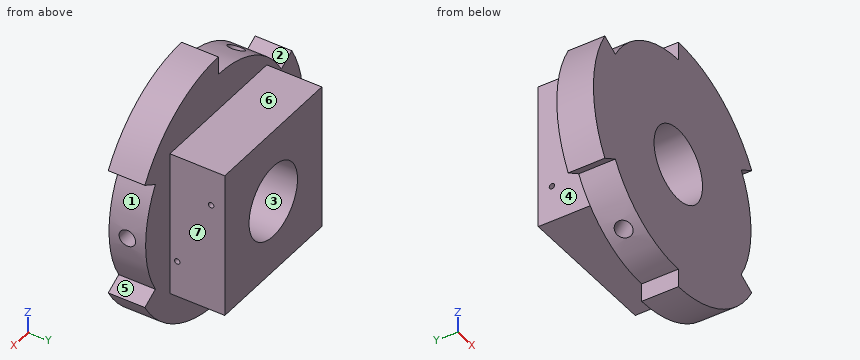
```python
from build123d import *

# Parameters (mm, degrees)
SKETCH1_R           = 30
BOSS_EXTRUDE3_DEPTH = 10
SKETCH2_R           = 2.25
CUT_EXTRUDE1_DEPTH  = 25
CIRPATTERN1_COUNT   = 3
SKETCH3_W           = 40
SKETCH3_H           = 40
BOSS_EXTRUDE4_DEPTH = 15
SKETCH5_R           = 10
CUT_EXTRUDE5_DEPTH  = 25
SKETCH4_R           = 0.75
CUT_EXTRUDE6_DEPTH  = 6
CIRPATTERN2_COUNT   = 2


with BuildPart() as part:
    # Sketch1 → Boss-Extrude3 (new body)
    with BuildSketch(Plane(origin=(0, 0, 0), x_dir=(1, 0, 0), z_dir=(0, 1, 0))):
        with BuildLine():
            Line((-25.980762114, 15), (-30.310889132, 17.5))
            ThreePointArc((-30.310889132, 17.5), (-35, 0), (-30.310889132, -17.5))
            Line((-30.310889132, -17.5), (-25.980762114, -15))
            ThreePointArc((-25.980762114, -15), (-30, 0), (-25.980762114, 15))
        make_face()
        Circle(SKETCH1_R)
        with BuildLine():
            Line((0, 35), (0, 30))
            ThreePointArc((0, 30), (15, 25.980762114), (25.980762114, 15))
            Line((25.980762114, 15), (30.310889132, 17.5))
            ThreePointArc((30.310889132, 17.5), (17.5, 30.310889132), (0, 35))
        make_face()
        with BuildLine():
            ThreePointArc((25.980762114, -15), (15, -25.980762114), (0, -30))
            Line((0, -30), (0, -35))
            ThreePointArc((0, -35), (17.5, -30.310889132), (30.310889132, -17.5))
            Line((30.310889132, -17.5), (25.980762114, -15))
        make_face()
    extrude(amount=BOSS_EXTRUDE3_DEPTH)

    # Sketch2 → Cut-Extrude1 (cut)
    with BuildSketch(Plane(origin=(40, 0, 0), x_dir=(0, 0, -1), z_dir=(1, 0, 0))):
        with Locations((0, 5)):
            Circle(SKETCH2_R)
    cut_extrude1 = extrude(amount=-CUT_EXTRUDE1_DEPTH, mode=Mode.SUBTRACT)

    # CirPattern1: Cut-Extrude1 ×3 about axis
    cirpattern1_axis = Axis((0, 0, 0), (0, 1, 0))
    for i in range(1, CIRPATTERN1_COUNT):
        add(cut_extrude1.rotate(cirpattern1_axis, i * 360 / CIRPATTERN1_COUNT), mode=Mode.SUBTRACT)

    # Sketch3 → Boss-Extrude4 (add)
    with BuildSketch(Plane(origin=(0, 10, 0), x_dir=(1, 0, 0), z_dir=(0, 1, 0))):
        Rectangle(SKETCH3_W, SKETCH3_H)
    extrude(amount=BOSS_EXTRUDE4_DEPTH)

    # Sketch5 → Cut-Extrude5 (cut)
    with BuildSketch(Plane(origin=(0, 25, 0), x_dir=(1, 0, 0), z_dir=(0, 1, 0))):
        with Locations(Location((0, 0, 0), (0, 0, 270))):
            Circle(SKETCH5_R)
    extrude(amount=-CUT_EXTRUDE5_DEPTH, mode=Mode.SUBTRACT)

    # Sketch4 → Cut-Extrude6 (cut)
    with BuildSketch(Plane(origin=(20, 0, 0), x_dir=(0, 0, -1), z_dir=(1, 0, 0))):
        with Locations((-10, 21.25)):
            Circle(SKETCH4_R)
        with Locations((10, 12)):
            Circle(SKETCH4_R)
    cut_extrude6 = extrude(amount=-CUT_EXTRUDE6_DEPTH, mode=Mode.SUBTRACT)

    # CirPattern2: Cut-Extrude6 ×2 about axis
    cirpattern2_axis = Axis((0, -28.284271247, 0), (0, 1, 0))
    for i in range(1, CIRPATTERN2_COUNT):
        add(cut_extrude6.rotate(cirpattern2_axis, i * 360 / CIRPATTERN2_COUNT), mode=Mode.SUBTRACT)


solid = part.part
```
Here's how the part is built. I have some questions about the finished solid (model axes, mm). Face numbers are marked on the shaded views. A direction names the side the tool comes from. Give positions to 0.01 mm unless a question says otherwise; leave off trailing zeros. Order: outer loops, then holes, each group sorted by start corner. A loop starts at its lowest first (then second) coordinate and runs counter-clockwise, first axis right, second up. Notation, with made-up numbers: M -13,1.25 L 3,1.25 A9 cw 3,8.25 Z; hole C 35,88.25 d7. An arc over 180 degrees is marked long. Use a Markdown table: item, result. Add a question column.
1. I need wall thicknesses on probe 1 along Y at (x, z) = (-17.15, 10); probe 2 along X at (y, z) = (14.75, 0); probe 3 along X at (y, z) = (3.5, -16). Which ranges of each line are inside material? Lowest first, please. Write a range as from..to.
2. If we mould it in two halves opening along Z, with no side actions, what happens to the marked faces 1, 2, 3 and 4? For each: +Z half, -Z half, draft (parallel to the pull), parting line (faces both ways), or undercut.
3. Suppose I cut it at C-C (x = -3). List the corners of the cut face in (y, z) for me, and give its area (3 significant figures).
4. Suppose I cut it at D-D (z = 16). Give the number of separate pieces and of enclosed holes in the cut face, and give its area (3 significant figures).
5. Suppose I cut it at A-A (z = 0). List the corners of the cut face in (x, y) for me.
6. For pin 1 Ø10 at (x, z) = (7, 16) entering from -Y; pin 2 Ø3.5 at (y, z) = (5, 0) entering from +X; pin 3 Ø12 at (x, y) = (-7.5, 20.5) entering from -Z; pin 4 Ø7.5 at (y, z) = (21, 5) entering from +X, each with a flat end and sliding along its axis, tell me the tip position at first contact or that it passes through.
7. Suppose I cut it at B-B (y = 17.25). List the corners of the cut face in (x, z) for me, and give its area (3 significant figures).
8. On a 3-axis mill with a long thin cutter (end or side, diameter ignored), from which of +Z, -Z, +X, -X, +Y, -Y can I reach the whole of each face in a straight line? I mean the marked faces 5, 6 and 7. Say none if no direction works.
Results list:
| question | item | result |
|---|---|---|
| 1 | probe 1 | y = 0..11.25, 12.75..25 |
| 1 | probe 2 | x = -20..-10, 10..20 |
| 1 | probe 3 | x = -31.13..-27.71, -25.38..-11.17, -7.3..27.71 |
| 2 | face 1 | undercut |
| 2 | face 2 | +Z half |
| 2 | face 3 | undercut |
| 2 | face 4 | draft |
| 3 | outline | M 0,-29.85 L 10,-29.85 L 10,-20 L 25,-20 L 25,-9.54 L 0,-9.54 Z; M 0,9.54 L 25,9.54 L 25,20 L 10,20 L 10,29.85 L 0,29.85 Z |
| 3 | area | 720 mm² |
| 4 | separate pieces | 2 |
| 4 | enclosed holes | 1 |
| 4 | area | 1,150 mm² |
| 5 | outline | M -35,0 L -10,0 L -10,25 L -20,25 L -20,10 L -35,10 Z; M 10,0 L 30,0 L 30,2.75 L 15,2.75 L 15,7.25 L 30,7.25 L 30,10 L 20,10 L 20,25 L 10,25 Z |
| 6 | pin 1 | stops at y = 0 |
| 6 | pin 2 | stops at x = 15 |
| 6 | pin 3 | stops at z = -20 |
| 6 | pin 4 | stops at x = 20 |
| 7 | outline | M -20,-20 L 20,-20 L 20,20 L -20,20 Z; hole C 0,0 d20 |
| 7 | area | 1,290 mm² |
| 8 | face 5 | +X, +Y, -Y |
| 8 | face 6 | +Z, +X, -X, +Y |
| 8 | face 7 | +Z, -Z, +X, +Y |
